The listing builds one solid part. Answer for the finished solid, in the listing's coordinates (mm). A direction names the side the tool comes from. Give positions to 0.01 mm unless a question says otherwise; leave off trailing zeros. Write each loop counter-clockwise with the first axis right and the second up, starting at its lowest first coordinate (ties: lowest second). Pieces come first, ordered by that corner, then holes. Notation, with made-up numbers: (88.5, 63) - (146.5, 63) arc R21 cw to (146.5, 99) - close; hole circle Ø7 at (-22, 5). An arc over 180 degrees is marked (long way). Return JSON: item names as keys, results as strings.
from build123d import *
from build123d import SkipClean  # not in build123d's __all__

# Parameters (mm, degrees)
F0_R           = 6.35
F0_R_2         = 3.81
F1_DEPTH       = 12.7
F4_DEPTH       = 38.1
F5_DEPTH       = 25.4
F5_DEPTH_BACK  = 25.4
F6_W           = 13.8230553448
F6_H           = 5.08
F7_DEPTH       = 7.62
F7_DEPTH_BACK  = 15.24
F8_DEPTH       = 7.62
F9_DEPTH       = 7.62
F11_DEPTH      = 25.4
F12_DEPTH      = 5.08
F14_DEPTH      = 38.1
F15_DEPTH      = 25.4
F16_W          = 2.54
F16_H          = 9.144
F17_DEPTH      = 2.54
F18_W          = 2.54
F18_H          = 8.89
F19_DEPTH      = 2.54
F21_DEPTH      = 12.7
F21_DEPTH_BACK = 12.7


with BuildPart() as f1:
    # F0 (on Front) → F1 (new body)
    with BuildSketch(Plane.XZ):
        Circle(F0_R)
        Circle(F0_R_2, mode=Mode.SUBTRACT)
    extrude(amount=F1_DEPTH)

    # F3 (on Right) → F4 (join)
    with BuildSketch(Plane.YZ):
        Polygon((-2.54, -2.54), (-2.54, 0), (-2.54, 2.54), (-10.16, 2.54), (-10.16, 0), (-10.16, -2.54), align=None)
    extrude(amount=F4_DEPTH)

    # F0 (on Front) → F5 (cut, two sides)
    with BuildSketch(Plane.XZ) as f5_sk:
        Circle(F0_R_2)
    extrude(amount=F5_DEPTH, mode=Mode.SUBTRACT)
    extrude(f5_sk.sketch, amount=-F5_DEPTH_BACK, mode=Mode.SUBTRACT)

    # F6 (on face) → F7 (join, two sides)
    with BuildSketch(Plane.XZ.offset(10.16)) as f7_sk:
        with Locations((31.1884723276, 0)):
            Rectangle(F6_W, F6_H)
    extrude(amount=F7_DEPTH)
    extrude(f7_sk.sketch, amount=-F7_DEPTH_BACK)

    # F8 (add): a face of the model
    f8_faces = [f1.faces().sort_by_distance(p)[0] for p in [
        (24.2769446552, -13.97, 0),
    ]]
    extrude(f8_faces, amount=F8_DEPTH)

    # F9 (add): a face of the model
    f9_faces = [f1.faces().sort_by_distance(p)[0] for p in [
        (24.2769446552, 1.27, 0),
    ]]
    extrude(f9_faces, amount=F9_DEPTH)

    # F10 (on face) → F11 (cut)
    with BuildSketch(Plane.XY.offset(2.54)):
        with BuildLine():
            ThreePointArc((25.9835010893, -17.78), (20.2469210754, -15.2836758241), (16.6569446552, -10.16))
            Line((16.6569446552, -10.16), (16.6569446552, -17.78))
            Line((16.6569446552, -17.78), (25.9835010893, -17.78))
        make_face()
        with BuildLine():
            Line((16.6569446552, 5.08), (16.6569446552, -2.54))
            ThreePointArc((16.6569446552, -2.54), (20.2469210754, 2.5836758241), (25.9835010893, 5.08))
            Line((25.9835010893, 5.08), (16.6569446552, 5.08))
        make_face()
        with BuildLine():
            Line((38.1, 5.08), (29.1083570088, 5.08))
            ThreePointArc((29.1083570088, 5.08), (34.4861831348, 2.8651480918), (38.1, -1.6919244863))
            Line((38.1, -1.6919244863), (38.1, 5.08))
        make_face()
        with BuildLine():
            Line((38.1, -17.78), (38.1, -11.0080755137))
            ThreePointArc((38.1, -11.0080755137), (34.4861831348, -15.5651480918), (29.1083570088, -17.78))
            Line((29.1083570088, -17.78), (38.1, -17.78))
        make_face()
    extrude(amount=-F11_DEPTH, mode=Mode.SUBTRACT)

    # F10 (on face) → F12 (join)
    with BuildSketch(Plane.XY.offset(2.54)):
        with BuildLine():
            ThreePointArc((38.1, -11.0080755137), (39.0822231303, -6.35), (38.1, -1.6919244863))
            Line((38.1, -1.6919244863), (38.1, -11.0080755137))
        make_face()
    with SkipClean():  # cleaning this boolean's faces spoils the solid; the shape is the same uncleaned
        extrude(amount=-F12_DEPTH)

    # F13 (on Top) → F14 (join)
    with BuildSketch(Plane.XY):
        Polygon((2.54, -2.54), (0, -2.54), (-2.54, -2.54), (-2.54, -10.16), (0, -10.16), (2.54, -10.16), align=None)
    extrude(amount=F14_DEPTH)

    # F0 (on Front) → F15 (cut)
    with BuildSketch(Plane.XZ):
        Circle(F0_R_2)
    extrude(amount=F15_DEPTH, mode=Mode.SUBTRACT)

    # F16 (on face) → F17 (cut)
    with BuildSketch(Plane(origin=(0, -2.54, 0), x_dir=(-1, 0, 0), z_dir=(0, 1, 0))):
        with Locations((-1.27, 33.528)):
            Rectangle(F16_W, F16_H)
        with Locations((1.27, 33.528)):
            Rectangle(F16_W, F16_H)
    extrude(amount=-F17_DEPTH, mode=Mode.SUBTRACT)

    # F18 (on face) → F19 (cut)
    with BuildSketch(Plane.XZ.offset(10.16)):
        with Locations((-1.27, 33.655)):
            Rectangle(F18_W, F18_H)
        with Locations((1.27, 33.655)):
            Rectangle(F18_W, F18_H)
    extrude(amount=-F19_DEPTH, mode=Mode.SUBTRACT)

    # F20 (on Front) → F21 (join, two sides)
    with BuildSketch(Plane.XZ) as f21_sk:
        with BuildLine():
            ThreePointArc((0, 34.1351066256), (2.6940768363, 35.2510297892), (3.81, 37.9451066256))
            ThreePointArc((3.81, 37.9451066256), (-2.6940768363, 40.6391834619), (0, 34.1351066256))
        make_face()
    extrude(amount=F21_DEPTH)
    extrude(f21_sk.sketch, amount=-F21_DEPTH_BACK)


solid = f1.part
Item 1: A cutting plane is placed at A-A on y = -9. Determine the outline of the cut face in (x, z).
Answer below:
{"outline": "circle Ø7.62 at (0, 37.95); (-2.54, 5.82) arc R6.35 ccw (long way) to (5.82, -2.54) - (38.77, -2.54) - (38.77, 2.54) - (5.82, 2.54) arc R6.35 ccw to (2.54, 5.82) - (2.54, 29.21) - (-2.54, 29.21) - close; hole circle Ø7.62 at (0, 0)"}
Item 2: A cutting plane is placed at C-C on z = 20. Determine the outline of the cut face in (x, y), then the cut area to 3 significant figures.
Answer below:
{"outline": "(-2.54, -10.16) - (2.54, -10.16) - (2.54, -2.54) - (-2.54, -2.54) - close", "area": "38.7 mm²"}
Item 3: A cutting plane is placed at B-B on z = 0. Determine the outline of the cut face in (x, y).
Answer below:
{"outline": "(-6.35, -12.7) - (-3.81, -12.7) - (-3.81, 0) - (-6.35, 0) - close; (3.81, -12.7) - (6.35, -12.7) - (6.35, -10.16) - (16.66, -10.16) arc R11.54 ccw to (25.98, -17.78) - (29.11, -17.78) arc R11.54 ccw to (29.11, 5.08) - (25.98, 5.08) arc R11.54 ccw to (16.66, -2.54) - (6.35, -2.54) - (6.35, 0) - (3.81, 0) - close"}
Item 4: A cutting plane is placed at D-D on x = 5. Determine the outline of the cut face in (y, z).
Answer below:
{"outline": "(-12.7, -3.91) - (0, -3.91) - (0, 3.91) - (-12.7, 3.91) - close"}
Item 5: Consider L1, parallel to Z at x = 0, y = -9; L2, parallel to Z at x = 0, y = -6; L3, parallel to Z at x = -2, y = -4.5. Determine where each line is inside the solid, lowest interval first.
Answer below:
{"L1": "z = -6.35 to -3.81, 3.81 to 29.21, 34.14 to 41.76", "L2": "z = -6.35 to -3.81, 3.81 to 41.76", "L3": "z = -6.03 to -3.24, 3.24 to 28.96, 34.7 to 41.19"}
Item 6: The mould has two halves that part along Z. Classify faces 6 (the face through (28, -17.78, 0)), 7 (the face through (-5.04, -6.26, -3.86)), 8 (the face through (26, -7, -2.54)), 9 (the face through (26, -7, 2.54)): +Z half, -Z half, draft (parallel to the pull), parting line (faces both ways), or undercut.
Answer below:
{"face 6": "draft", "face 7": "undercut", "face 8": "-Z half", "face 9": "+Z half"}
Item 7: Flat-ended cylindrical pins translate along their axes: P1, Ø10, axis at x = 0, z = -2.5, coming from the -Y side; P2, Ø12, axis at x = 16, y = -11.5, coming from the -Z side; P3, Ø10, axis at y = -9.5, z = 35.5, coming from the -X side; P4, Ø4.5, axis at x = 0, z = 0, coming from the +Y side. Find the tip coordinate at first contact, or state that the pin passes through.
Answer below:
{"P1": "stops at y = -12.7", "P2": "stops at z = -2.54", "P3": "stops at x = -3.81", "P4": "passes through"}
Item 8: For faces 1 (the face through (0, -4, 28.956)), 2 (the face through (3, -12.7, -3)), 3 (the face through (2.54, -6, 17)), 4 (the face through (3, 0, -3)), 5 (the face through (20.18, 2.53, 0.04)), determine the directions among +Z, -Z, +X, -X, +Y, -Y from which every point of the face is accessible in a straight line to the end or side of a thin tool.
Answer below:
{"face 1": "+X, -X, +Y", "face 2": "+Z, -Z, -X, -Y", "face 3": "+X, +Y, -Y", "face 4": "-Z, -X, +Y", "face 5": "+Z, -Z, +Y"}
